CAD build for the part. Positions are in the model's coordinates, mm. A direction names the side the tool comes from. Round coordinates to 2 decimals unless told otherwise and drop trailing zeros. Write each loop counter-clockwise with the first axis right and the second up, starting at its lowest first coordinate (ties: lowest second). Pieces come first, ordered by that corner, then holes. Notation, with made-up numbers: M 86,84 L 144,84 A18 cw 144,112 Z; hole C 19.25,-17.5 d9. An arc over 180 degrees is marked long. Write each question's results on one line, items separated by ' | '. Start each with the question number.
```python
from build123d import *

# Parameters (mm, degrees)
SKETCH_1_W            = 42
SKETCH_1_H            = 25.4
EXTRUDE_1_DEPTH       = 70
SKETCH_5_W            = 6
SKETCH_5_H            = 25.4
EXTRUDE_5_DEPTH       = 70
SKETCH_6_R            = 3.96875
CUT_EXTRUDE_2_DEPTH   = 83.61531335
FILLET_6_R            = 4
HOLE_WIZARD_10_32_1_D = 4.0386
FILLET_7_R            = 12.7
SKETCH_9_W            = 42
SKETCH_9_H            = 25
CUT_EXTRUDE_3_DEPTH   = 78.370278531


with BuildPart() as part:
    # 草圖1 → 填料-伸長1 (new body)
    with BuildSketch(Plane(origin=(0, 0, 0), x_dir=(1, 0, 0), z_dir=(0, 1, 0))):
        Rectangle(SKETCH_1_W, SKETCH_1_H)
    extrude(amount=EXTRUDE_1_DEPTH)

    # 草圖5 → 填料-伸長5 (add)
    with BuildSketch(Plane.XZ):
        with Locations((-18, 0)):
            Rectangle(SKETCH_5_W, SKETCH_5_H)
        with Locations((18, 0)):
            Rectangle(SKETCH_5_W, SKETCH_5_H)
    extrude(amount=EXTRUDE_5_DEPTH)

    # 草圖6 → 除料-伸長2 (cut, through all)
    with BuildSketch(Plane.ZY.offset(21)):
        with Locations((0, -57.3)):
            Circle(SKETCH_6_R)
    extrude(amount=-CUT_EXTRUDE_2_DEPTH, mode=Mode.SUBTRACT)

    # 圓角6
    fillet_6_edges = [part.edges().sort_by_distance(p)[0] for p in [
        (15, 0, 0),
        (-15, 0, 0),
    ]]
    fillet(fillet_6_edges, radius=FILLET_6_R)

    # #10-32 螺紋孔1 (through all)
    with Locations(Plane.XY.offset(12.7)):
        with Locations((0, 30), (0, 15)):
            Hole(HOLE_WIZARD_10_32_1_D / 2)

    # 圓角7
    fillet_7_edges = [part.edges().sort_by_distance(p)[0] for p in [
        (18, -70, 12.7),
        (18, -70, -12.7),
        (-18, -70, 12.7),
        (-18, -70, -12.7),
    ]]
    fillet(fillet_7_edges, radius=FILLET_7_R - 0.0001)  # a hair under: the kernel refuses the full size

    # 草圖9 → 除料-伸長3 (cut, through all)
    with BuildSketch(Plane.XY.offset(12.7)):
        with Locations((0, 57.5)):
            Rectangle(SKETCH_9_W, SKETCH_9_H)
    extrude(amount=-CUT_EXTRUDE_3_DEPTH, mode=Mode.SUBTRACT)


solid = part.part
```
1) Saw through at B-B, the plane y = 15. Write the cut outline in (x, z), plus the area to 3 significant figures.
2) Pull direction X, two halves, no side cores. Call faces 1 (the face through (-21, -12, 0)), 2 (the face through (21, -13, 0)), 3 (the face through (13.797, -1.141, 0.178)), 4 (the face through (0, 6, -12.7)): pulls with the +X half, pulls with the -X half, needs draft (parallel to the pull), parting line crosses it, or undercut.
3) 3-axis set-ups, long thin cutter, end or side, ignore diameter. For faces 5 (the face through (-15, -37, 0)), 6 (the face through (0.44, 13.03, -0.18)): which of +Z, -Z, +X, -X, +Y, -Y reach the whole face in a straight line?
4) Saw through at C-C, the plane y = -38. Write the cut outline in (x, z).
5) Saw through at D-D, the plane z = 8.5. Write the cut outline in (x, y).
6) Saw through at A-A, the plane x = 0. Write the cut outline in (y, z), plus the area to 3 significant figures.
7) Wall check: line 1 along Y through (x, z) = (0, -6); line 2 along X through (y, z) = (-50, -1.5); line 3 along Y through (x, z) = (7.5, 9.75). Give the ranges that are in metal, low to high. Write a range as from..to.
8) Drop flat-ended pins along their axis: pin 1 Ø3.5 at (x, y) = (0, 15) entering from -Z; pin 2 Ø10.5 at (y, z) = (-57.3, 0) entering from -X; pin 3 Ø4 at (x, z) = (1.5, 6.5) entering from -Y. Give the stop position or say it passes through.
Filled sheet:
1) outline: M -21,-12.7 L -2.02,-12.7 L -2.02,12.7 L -21,12.7 Z; M 2.02,-12.7 L 21,-12.7 L 21,12.7 L 2.02,12.7 Z | area: 964 mm^2
2) face 1: pulls with the -X half | face 2: pulls with the +X half | face 3: undercut | face 4: needs draft
3) face 5: +Z, -Z, -Y | face 6: +Z, -Z
4) outline: M -21,-12.7 L -15,-12.7 L -15,12.7 L -21,12.7 Z; M 15,-12.7 L 21,-12.7 L 21,12.7 L 15,12.7 Z
5) outline: M -21,-66.74 L -15,-66.74 L -15,-4 A4 cw -11,0 L 11,0 A4 cw 15,-4 L 15,-66.74 L 21,-66.74 L 21,45 L -21,45 Z; hole C 0,15 d4.04; hole C 0,30 d4.04
6) outline: M 0,-12.7 L 12.98,-12.7 L 12.98,12.7 L 0,12.7 Z; M 17.02,-12.7 L 27.98,-12.7 L 27.98,12.7 L 17.02,12.7 Z; M 32.02,-12.7 L 45,-12.7 L 45,12.7 L 32.02,12.7 Z | area: 938 mm^2
7) line 1: y = 0..12.98, 17.02..27.98, 32.02..45 | line 2: x = -21..-15, 15..21 | line 3: y = 0..45
8) pin 1: passes through | pin 2: stops at x = -21 | pin 3: stops at y = 0
